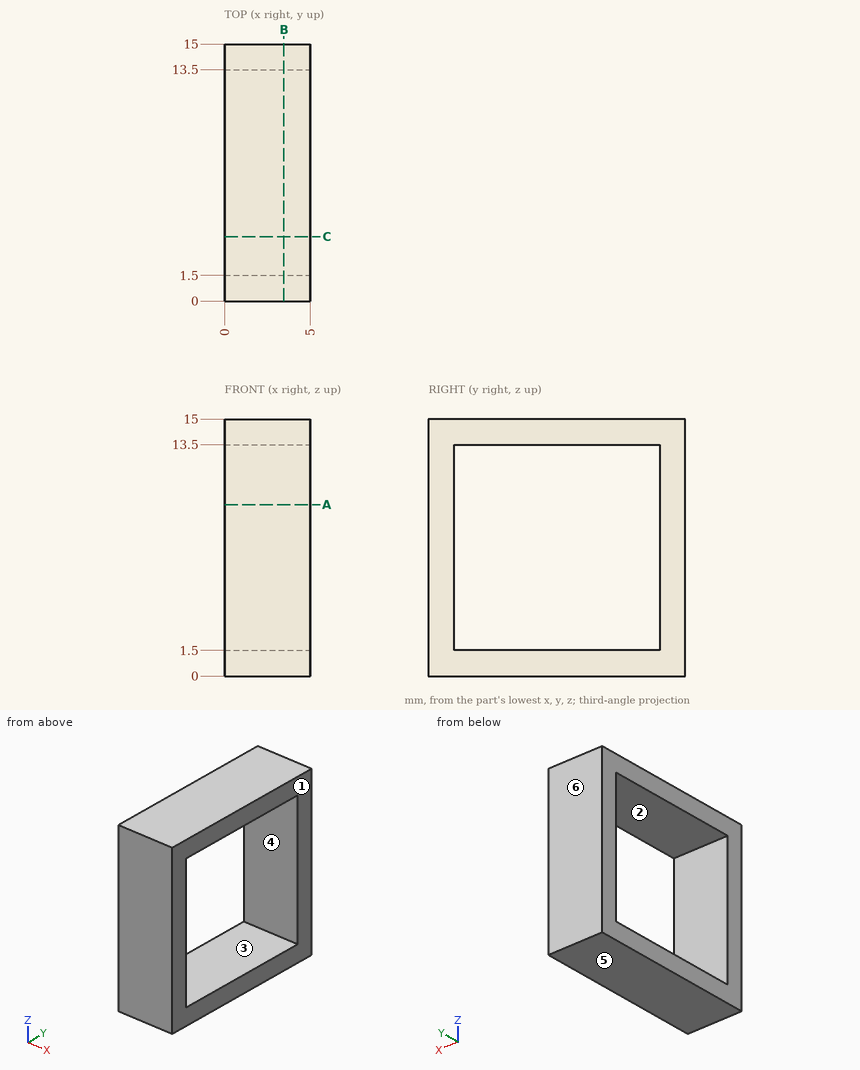
Verification items for this drawing (mm, ordinates from the low corner). A direction names the side the tool comes from. Give positions to 0.01 mm unless a question says otherwise; leave off trailing zeros. Loops run counter-clockwise (first coordinate to the right, second up) from the corner with the lowest first, then second, coordinate; pieces in that order, holes last. Notation, with made-up numbers: M 52,71 L 58,71 A11 cw 58,90 Z; hole C 84.5,60.25 d3. An arc over 180 degrees is marked long. Answer as a JSON object with one key per item and string values. Group by question number.
Q1. Access from +Z, -Z, +X, -X, +Y, -Y to the whole of each face (thin tool, end or side, straight path). Record for the marked faces 1 and 2.
Q2. Material ranges on line 1 along Y through (x, z) = (4.3, 11.75), recorded low to high. Write a range as [from, to].
Q3. Cross-section at A-A on z = 10. Record the cut outline in (x, y).
Q4. Release check for a two-part mould opening along Y. For the marked faces 3, 4, 5 and 6 record: released by +Y, released by -Y, zero draft, split by the parting line, or undercut.
Q5. Cross-section at B-B on x = 3.45. Record the cut outline in (y, z).
Evaluation:
{
 "1": {"face 1": "+Z, -Z, +X, +Y, -Y", "face 2": "+X, -X"},
 "2": {"line 1": "y = [0, 1.5], [13.5, 15]"},
 "3": {"outline": "M 0,0 L 5,0 L 5,1.5 L 0,1.5 Z; M 0,13.5 L 5,13.5 L 5,15 L 0,15 Z"},
 "4": {"face 3": "undercut", "face 4": "undercut", "face 5": "zero draft", "face 6": "released by +Y"},
 "5": {"outline": "M 0,0 L 15,0 L 15,15 L 0,15 Z; hole M 1.5,1.5 L 13.5,1.5 L 13.5,13.5 L 1.5,13.5 Z"}
}
